Check sheet for the modelled part. Datum: model origin and axes. Units: mm. Round coordinates to 2 decimals unless told otherwise and drop trailing zeros. Order: outer loops, then holes, each group sorted by start corner. A loop starts at its lowest first (then second) coordinate and runs counter-clockwise, first axis right, second up.
```python
from build123d import *

# Parameters (mm, degrees)
SKETCH_W        = 347
SKETCH_H        = 420
PAD_DEPTH       = 3
SKETCH001_R     = 1.75
POCKET_DEPTH    = 3.001
SKETCH002_R     = 2
SKETCH002_R_2   = 12
POCKET001_DEPTH = 5
SKETCH003_R     = 2
SKETCH003_W     = 29
SKETCH003_H     = 49
SKETCH003_W_2   = 13
SKETCH003_H_2   = 13
POCKET002_DEPTH = 3.001


with BuildPart() as part:
    # Sketch → Pad (new body)
    with BuildSketch(Plane.XZ):
        with Locations((173.5, 210)):
            Rectangle(SKETCH_W, SKETCH_H)
    extrude(amount=PAD_DEPTH)

    # Sketch001 (on Face6 of Pad) → Pocket (cut, through all)
    with BuildSketch(Plane.XZ.offset(3)):
        with Locations((45, 45)):
            Circle(SKETCH001_R)
        with Locations((302, 45)):
            Circle(SKETCH001_R)
        with Locations((302, 410)):
            Circle(SKETCH001_R)
        with Locations((45, 410)):
            Circle(SKETCH001_R)
    extrude(amount=-POCKET_DEPTH, mode=Mode.SUBTRACT)

    # Sketch002 (on Face5 of Pocket) → Pocket001 (cut)
    with BuildSketch(Plane.XZ.offset(3)):
        with Locations((25, 301)):
            Circle(SKETCH002_R)
        with Locations((25, 270)):
            Circle(SKETCH002_R)
        with Locations((56, 270)):
            Circle(SKETCH002_R)
        with Locations((56, 301)):
            Circle(SKETCH002_R)
        with Locations((40.5, 285.5)):
            Circle(SKETCH002_R_2)
        with BuildLine():
            ThreePointArc((37, 361), (34, 364), (31, 361))
            Line((31, 361), (31, 336))
            ThreePointArc((31, 336), (34, 333), (37, 336))
            Line((37, 361), (37, 336))
        make_face()
        with BuildLine():
            ThreePointArc((50, 361), (47, 364), (44, 361))
            Line((44, 361), (44, 336))
            ThreePointArc((44, 336), (47, 333), (50, 336))
            Line((50, 361), (50, 336))
        make_face()
    extrude(amount=-POCKET001_DEPTH, mode=Mode.SUBTRACT)

    # Sketch003 (on Face5 of Pocket001) → Pocket002 (cut, through all)
    with BuildSketch(Plane.XZ.offset(3)):
        with Locations((298.5, 84.5)):
            Circle(SKETCH003_R)
        with Locations((338.5, 84.5)):
            Circle(SKETCH003_R)
        with Locations((303.5, 24)):
            Circle(SKETCH003_R)
        with Locations((333.5, 24)):
            Circle(SKETCH003_R)
        with Locations((318.5, 84.5)):
            Rectangle(SKETCH003_W, SKETCH003_H)
        with Locations((318.5, 24)):
            Rectangle(SKETCH003_W_2, SKETCH003_H_2)
    extrude(amount=-POCKET002_DEPTH, mode=Mode.SUBTRACT)


solid = part.part
```
Item 1: Sectioned sample at A-A (z = 102.5). Record the cut outline in (x, y).
Answer:
outline: (0, -3) - (304, -3) - (304, 0) - (0, 0) - close; (333, -3) - (347, -3) - (347, 0) - (333, 0) - close
Item 2: Sectioned sample at C-C (z = 285.5). Record the cut outline in (x, y), and give its area (3 significant figures).
Answer:
outline: (0, -3) - (28.5, -3) - (28.5, 0) - (0, 0) - close; (52.5, -3) - (347, -3) - (347, 0) - (52.5, 0) - close
area: 969 mm2
Item 3: Scan lines: line 1 along X through (y, z) = (-1.4, 301); line 2 along Z through (x, y) = (298.5, -2.2); line 3 along Z through (x, y) = (56, -2.3). Record each from-to range of solid material in increasing order.
Answer:
line 1: x = 0 to 23, 27 to 54, 58 to 347
line 2: z = 0 to 82.5, 86.5 to 420
line 3: z = 0 to 268, 272 to 299, 303 to 420
Item 4: Release check for a two-part mould opening along X. For faces 1 (the cylindrical face through (37.899, -1.521, 273.785)), 2 (the flat face through (171, -3, 213)) record: released by +X, released by -X, zero draft, split by the parting line, or undercut.
Answer:
face 1: undercut
face 2: zero draft
Item 5: Sectioned sample at B-B (y = -1.9). State how many separate pieces and enclosed holes the cut face has, and give its area (3 significant figures).
Answer:
separate pieces: 1
enclosed holes: 17
area: 143,000 mm2
